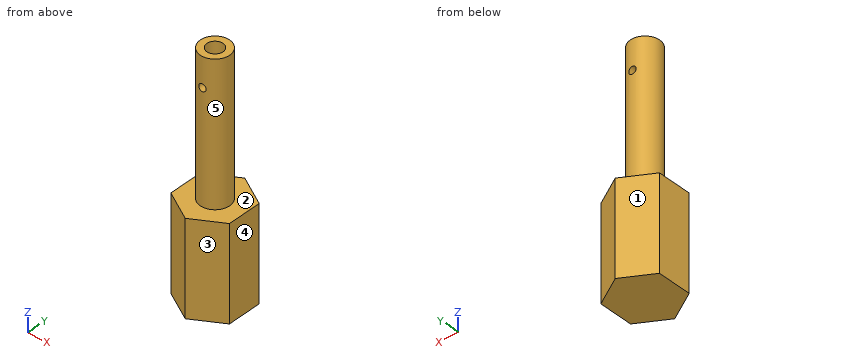
```python
from build123d import *

# Parameters (mm, degrees)
BOSS_EXTRUDE1_DEPTH            = 20.32
SKETCH2_R                      = 3.175
BOSS_EXTRUDE2_DEPTH            = 30.48
F_3_5_3_5_DIAMETER_HOLE1_D     = 3.5
F_3_5_3_5_DIAMETER_HOLE1_DEPTH = 25.4
F_3_5_3_5_DIAMETER_HOLE1_TIP   = 1.051506083
F_1_16_0_0625_DIAMETER_HOLE1_D = 1.5875


with BuildPart() as part:
    # Sketch1 → Boss-Extrude1 (new body)
    with BuildSketch(Plane.XY):
        Polygon((0, 7.332348419), (-6.35, 3.666174209), (-6.35, -3.666174209), (0, -7.332348419), (6.35, -3.666174209), (6.35, 3.666174209), align=None)
    extrude(amount=BOSS_EXTRUDE1_DEPTH)

    # Sketch2 → Boss-Extrude2 (add)
    with BuildSketch(Plane.XY.offset(20.32)):
        Circle(SKETCH2_R)
    extrude(amount=BOSS_EXTRUDE2_DEPTH)

    # Ø3.5 (3.5) Diameter Hole1
    with Locations(Plane.XY.offset(50.8)):
        with Locations((0, 0)):
            Hole(F_3_5_3_5_DIAMETER_HOLE1_D / 2, depth=F_3_5_3_5_DIAMETER_HOLE1_DEPTH)
            with Locations((0, 0, -(F_3_5_3_5_DIAMETER_HOLE1_DEPTH + F_3_5_3_5_DIAMETER_HOLE1_TIP / 2))):  # 118° drill point
                Cone(0, F_3_5_3_5_DIAMETER_HOLE1_D / 2, F_3_5_3_5_DIAMETER_HOLE1_TIP, mode=Mode.SUBTRACT)

    # 1/16 (0.0625) Diameter Hole1 (through all)
    with Locations(Plane(origin=(0, 7.62, 0), x_dir=(1, 0, 0), z_dir=(0, 1, 0))):
        with Locations((0, -44.45)):
            Hole(F_1_16_0_0625_DIAMETER_HOLE1_D / 2)


solid = part.part
```
Model file for the job. Use its own axes, mm. Face numbers are marked on the shaded views. A direction names the side the tool comes from. Coordinates: 2 decimals unless noted, no trailing zeros. Write each loop counter-clockwise with the first axis right and the second up, starting at its lowest first coordinate (ties: lowest second). Pieces come first, ordered by that corner, then holes. Notation, with made-up numbers: (67, 55.25) - (111, 55.25) arc R26 cw to (111, 89.25) - close; hole circle Ø4 at (-28.75, 72). An arc over 180 degrees is marked (long way). Use a Markdown table: item, result. Add a question column.
Item 1: 3-axis set-ups, long thin cutter, end or side, ignore diameter. For the marked faces 1 and 2: which of +Z, -Z, +X, -X, +Y, -Y reach the whole face in a straight line?
Item 2: Drop flat-ended pins along their axis: pin 1 (3 mm diameter, centred on x = 4, y = 6, fed in from +Z); pin 2 (1.5 mm diameter, centred on y = 2, z = 37, fed in from -X); pin 3 (6 mm diameter, centred on x = 2.5, z = 18, fed in from +Y). Give the stop position or say it passes through.
Item 3: Band-saw the part on B-B, the plane z = 36.5. Write the cut outline in (x, y) (3 decimals).
Item 4: Band-saw the part on C-C, the plane y = -5. Write the cut outline in (x, z).
Item 5: Band-saw the part on A-A, the plane z = 44.45. Write the cut outline in (x, y) (3 decimals).
Item 6: Two-plate mould, pull along Y, no slides. Class the marked faces 3, 4 and 5: pulls with the +Y half, pulls with the -Y half, needs draft (parallel to the pull), parting line crosses it, or undercut.
Item 7: Drill centre lines: line 1 along Z through (x, y) = (0, -2.7); line 2 along Y through (x, z) = (0, 33) (3 decimals); line 3 along Y through (x, z) = (-1.25, 44). Where is each one in solid material? Low to high.
A:
| question | item | result |
|---|---|---|
| 1 | face 1 | +Z, -Z, -X, +Y |
| 1 | face 2 | +Z |
| 2 | pin 1 | stops at z = 20.32 |
| 2 | pin 2 | stops at x = -2.92 |
| 2 | pin 3 | stops at y = 7.33 |
| 3 | outline | circle Ø6.35 at (0, 0); hole circle Ø3.5 at (0, 0) |
| 4 | outline | (-4.04, 0) - (4.04, 0) - (4.04, 20.32) - (-4.04, 20.32) - close |
| 5 | outline | (-0.794, -3.074) - (-0.794, -1.56) arc R1.75 cw to (-0.794, 1.56) - (-0.794, 3.074) arc R3.175 ccw to start; (0.794, -3.074) arc R3.175 ccw to (0.794, 3.074) - (0.794, 1.56) arc R1.75 cw to (0.794, -1.56) - close |
| 6 | face 3 | pulls with the -Y half |
| 6 | face 4 | needs draft |
| 6 | face 5 | parting line crosses it |
| 7 | line 1 | z = 0 to 43.66, 45.24 to 50.8 |
| 7 | line 2 | y = -3.175 to -1.75, 1.75 to 3.175 |
| 7 | line 3 | y = -2.92 to -1.22, 1.22 to 2.92 |
